Part model, mm, in its own coordinate system. Coordinates: 2 decimals unless noted, no trailing zeros. Loops run counter-clockwise (first coordinate to the right, second up) from the corner with the lowest first, then second, coordinate; pieces in that order, holes last. Notation, with made-up numbers: M 52.5,-9.75 L 102.5,-9.75 A32 cw 102.5,25.25 Z; hole C 74.25,62.25 d10. An arc over 180 degrees is marked long. Use a Markdown table: item, result. Add a question column.
1) Wall check: probe 1 along Y at (x, z) = (25.5, 3); probe 2 along X at (y, z) = (95, 4.2). Give the ranges that are in metal, low to high. Write a range as from..to.
2) Band-saw the part on B-B (y = 80.5). List the corners of the cut face in (x, z).
3) Pin check, flat tips, straight feed: pin 1 Ø3 at (y, z) = (-35.5, 2.5) entering from +X; pin 2 Ø1 at (x, z) = (-31.5, 2) entering from -Y; pin 3 Ø2.5 at (x, z) = (178, 2.5) entering from +Y. Stop position of each tip, or through.
4) Band-saw the part on A-A (x = -24.5). List the corners of the cut face in (y, z).
from build123d import *

# Parameters (mm, degrees)
SKETCH1_W           = 350
SKETCH1_H           = 199
BOSS_EXTRUDE1_DEPTH = 5
SKETCH2_W           = 5
SKETCH2_H           = 25
BOSS_EXTRUDE2_DEPTH = 5
SKETCH3_W           = 25
SKETCH3_H           = 5
BOSS_EXTRUDE3_DEPTH = 5


with BuildPart() as part:
    # Sketch1 → Boss-Extrude1 (new body)
    with BuildSketch(Plane.XY):
        Rectangle(SKETCH1_W, SKETCH1_H)
    extrude(amount=BOSS_EXTRUDE1_DEPTH)

    # Sketch2 → Boss-Extrude2 (add)
    with BuildSketch(Plane(origin=(175, 0, 0), x_dir=(0, 0, -1), z_dir=(1, 0, 0))):
        with Locations((-2.5, 61.5)):
            Rectangle(SKETCH2_W, SKETCH2_H)
        with Locations((-2.5, 20.5)):
            Rectangle(SKETCH2_W, SKETCH2_H)
        with Locations((-2.5, -20.5)):
            Rectangle(SKETCH2_W, SKETCH2_H)
        with Locations((-2.5, -61.5)):
            Rectangle(SKETCH2_W, SKETCH2_H)
    boss_extrude2 = extrude(amount=BOSS_EXTRUDE2_DEPTH)

    # Mirror1: Boss-Extrude2 across plane
    add(boss_extrude2.mirror(Plane(origin=(0, 0, 0), x_dir=(0, 0, 1), z_dir=(1, 0, 0))))

    # Sketch3 → Boss-Extrude3 (add)
    with BuildSketch(Plane(origin=(0, 99.5, 0), x_dir=(1, 0, 0), z_dir=(0, 1, 0))):
        with Locations((-112.5, -2.5)):
            Rectangle(SKETCH3_W, SKETCH3_H)
        with Locations((-56.25, -2.5)):
            Rectangle(SKETCH3_W, SKETCH3_H)
        with Locations((0, -2.5)):
            Rectangle(SKETCH3_W, SKETCH3_H)
        with Locations((56.25, -2.5)):
            Rectangle(SKETCH3_W, SKETCH3_H)
        with Locations((112.5, -2.5)):
            Rectangle(SKETCH3_W, SKETCH3_H)
    boss_extrude3 = extrude(amount=BOSS_EXTRUDE3_DEPTH)

    # Mirror2: Boss-Extrude3 across plane
    add(boss_extrude3.mirror(Plane.ZX))


solid = part.part
Entries:
| question | item | result |
|---|---|---|
| 1 | probe 1 | -99.5..99.5 |
| 1 | probe 2 | -175..175 |
| 2 | outline | M -175,0 L 175,0 L 175,5 L -175,5 Z |
| 3 | pin 1 | x = 175 |
| 3 | pin 2 | y = -99.5 |
| 3 | pin 3 | y = 74 |
| 4 | outline | M -99.5,0 L 99.5,0 L 99.5,5 L -99.5,5 Z |
